Geometry: final body of the model. Coordinates: model frame, mm. A direction names the side the tool comes from. Give positions to 0.01 mm unless a question says otherwise; leave off trailing zeros. Loops run counter-clockwise (first coordinate to the right, second up) from the corner with the lowest first, then second, coordinate; pieces in that order, holes last. Notation, with made-up numbers: M 69,14.5 L 90,14.5 A17 ccw 90,19.5 Z; hole C -1,18.25 d5. An arc over 180 degrees is marked long. One line per question, with ' | ' between items. Start each with the question number.
from build123d import *

# Parameters (mm, degrees)
BOSS_EXTRUDE1_DEPTH = 7.5
SKETCH2_R           = 10
BOSS_EXTRUDE2_DEPTH = 5


with BuildPart() as part:
    # Sketch1 → Boss-Extrude1 (new body)
    with BuildSketch(Plane(origin=(0, 0, 0), x_dir=(1, 0, 0), z_dir=(0, 1, 0))):
        with BuildLine():
            Line((-6, 34.481879299), (-6, 8))
            ThreePointArc((-6, 8), (-8.660254038, 5), (-9.92820323, 1.196152423))
            Line((-9.92820323, 1.196152423), (-32.862183443, -12.044787227))
            ThreePointArc((-32.862183443, -12.044787227), (-30.310889132, -17.5), (-26.862183443, -22.437092072))
            Line((-26.862183443, -22.437092072), (-3.92820323, -9.196152423))
            ThreePointArc((-3.92820323, -9.196152423), (0, -10), (3.92820323, -9.196152423))
            Line((3.92820323, -9.196152423), (26.862183443, -22.437092072))
            ThreePointArc((26.862183443, -22.437092072), (30.310889132, -17.5), (32.862183443, -12.044787227))
            Line((32.862183443, -12.044787227), (9.92820323, 1.196152423))
            ThreePointArc((9.92820323, 1.196152423), (8.660254038, 5), (6, 8))
            Line((6, 8), (6, 34.481879299))
            ThreePointArc((6, 34.481879299), (0, 35), (-6, 34.481879299))
        make_face()
    extrude(amount=BOSS_EXTRUDE1_DEPTH)

    # Sketch2 → Boss-Extrude2 (add)
    with BuildSketch(Plane(origin=(0, 7.5, 0), x_dir=(1, 0, 0), z_dir=(0, 1, 0))):
        with Locations(Location((0, 0, 0), (0, 0, 53.130102354))):
            Circle(SKETCH2_R)
    extrude(amount=BOSS_EXTRUDE2_DEPTH)

    # Sketch3 → Cut-Revolve1 (revolve, cut)
    with BuildSketch(Plane.XY):
        Polygon((0, 0), (0, 12.5), (3, 12.5), (3, 1.732050808), (6, 0), align=None)
    revolve(axis=Axis((0, 0, 0), (0, 1, 0)), mode=Mode.SUBTRACT)


solid = part.part
Q1. Draft query along X for faces 1 (the flat face through (5, 0, 4)), 2 (the flat face through (21.56, 3.7, 5.52)), 3 (the flat face through (-15.56, 3.7, 15.91)), 4 (the conical face through (-0.691, 1.624, 3.112)). Return one class per face: released by +X, released by -X, zero draft, split by the parting line, or undercut.
Q2. Set-up query: faces 5 (the cylindrical face through (0, 4, -35)), 6 (the flat face through (15.23, 3.7, 15.72)), 7 (the cylindrical face through (30.27, 3.7, 17.57)), 8 (the flat face through (6, 4, -21)), 9 (the flat face through (-6, 4, -21)). Return all of +Z, -Z, +X, -X, +Y, -Y with unobstructed straight access to the full face (end or side cutting, diameter ignored); none if empty.
Q3. Section D-D, the plane z = 7.5. Output: boundary loops of the cut face in (x, y), plus the area to 3 significant figures.
Q4. Section A-A, the plane x = 0. Output: boundary loops of the cut face in (y, z), plus the area to 3 significant figures.
Q5. Section C-C, the plane y = 3.75. Output: boundary loops of the cut face in (x, z).
Q6. Contact query for flat-ended pins moving along their axis: pin 1 (5 mm diameter, centred on y = 7, z = -23.5, fed in from -X); pin 2 (1 mm diameter, centred on y = 2, z = 16, fed in from +X); pin 3 (1 mm diameter, centred on y = 1.5, z = -26.5, fed in from +X); pin 4 (5.5 mm diameter, centred on x = 0, z = 0, fed in from -Y). Output: stop coordinate, or through.
Q7. Section B-B, the plane z = 0. Output: boundary loops of the cut face in (x, y), plus the area to 3 significant figures.
Q8. Material intervals for L1, parallel to Z at x = 0, y = 7.25; L2, parallel to X at y = 9.5, z = 0, sorted ascending.
Model answer:
1) face 1: zero draft | face 2: released by +X | face 3: undercut | face 4: undercut
2) face 5: -Z, +Y, -Y | face 6: +Z, +Y, -Y | face 7: +Z, +X, +Y, -Y | face 8: -Z, +X, +Y, -Y | face 9: -Z, -X, +Y, -Y
3) outline: M -24.99,0 L 24.99,0 L 24.99,7.5 L 6.61,7.5 L 6.61,12.5 L -6.61,12.5 L -6.61,7.5 L -24.99,7.5 Z | area: 441 mm^2
4) outline: M 0,-35 L 7.5,-35 L 7.5,-10 L 12.5,-10 L 12.5,-3 L 1.73,-3 L 0,-6 Z; M 0,6 L 1.73,3 L 12.5,3 L 12.5,10 L 0,10 Z | area: 357 mm^2
5) outline: M -32.86,12.04 L -9.93,-1.2 A10 ccw -6,-8 L -6,-34.48 A35 ccw 6,-34.48 L 6,-8 A10 ccw 9.93,-1.2 L 32.86,12.04 A35 ccw 26.86,22.44 L 3.93,9.2 A10 ccw -3.93,9.2 L -26.86,22.44 A35 ccw Z; hole C 0,0 d6
6) pin 1: stops at x = -6 | pin 2: stops at x = 31.38 | pin 3: stops at x = 6 | pin 4: passes through
7) outline: M -12,0 L -6,0 L -3,1.73 L -3,12.5 L -10,12.5 L -10,7.5 L -12,7.5 Z; M 3,1.73 L 6,0 L 12,0 L 12,7.5 L 10,7.5 L 10,12.5 L 3,12.5 Z | area: 200 mm^2
8) L1: z = -35 to -3, 3 to 10 | L2: x = -10 to -3, 3 to 10
